from build123d import *

# Parameters (mm, degrees)
EXTRUDE_1_DEPTH = 2
SKETCH_2_R      = 2.5
EXTRUDE_2_DEPTH = 30


with BuildPart() as part:
    # 草图1 → 凸台-拉伸1 (new body)
    with BuildSketch(Plane(origin=(0, 0, 0), x_dir=(1, 0, 0), z_dir=(0, 1, 0))):
        with BuildLine():
            Line((64.772727273, 118.409090909), (138.257575758, 118.409090909))
            Line((138.257575758, 118.409090909), (138.257575758, 143.409090909))
            ThreePointArc((138.257575758, 143.409090909), (141.186507946, 150.480158721), (148.257575758, 153.409090909))
            Line((148.257575758, 153.409090909), (153.257575758, 153.409090909))
            ThreePointArc((153.257575758, 153.409090909), (160.328643569, 150.480158721), (163.257575758, 143.409090909))
            Line((163.257575758, 143.409090909), (163.257575758, 118.409090909))
            Line((163.257575758, 118.409090909), (200, 118.409090909))
            Line((200, 118.409090909), (200, 0))
            Line((200, 0), (0, 0))
            Line((0, 0), (0, 118.409090909))
            Line((0, 118.409090909), (39.772727273, 118.409090909))
            Line((39.772727273, 118.409090909), (39.772727273, 143.409090909))
            ThreePointArc((39.772727273, 143.409090909), (42.701659461, 150.480158721), (49.772727273, 153.409090909))
            Line((49.772727273, 153.409090909), (54.772727273, 153.409090909))
            ThreePointArc((54.772727273, 153.409090909), (61.843795085, 150.480158721), (64.772727273, 143.409090909))
            Line((64.772727273, 143.409090909), (64.772727273, 118.409090909))
        make_face()
    extrude(amount=EXTRUDE_1_DEPTH)

    # 草图2 → 凸台-拉伸2 (add)
    with BuildSketch(Plane(origin=(0, 2, 0), x_dir=(1, 0, 0), z_dir=(0, 1, 0))):
        with Locations(Location((52.11924037, 143.695636013, 0), (0, 0, 90))):
            Circle(SKETCH_2_R)
        with Locations(Location((151.328174324, 143.695636013, 0), (0, 0, 90))):
            Circle(SKETCH_2_R)
    extrude(amount=EXTRUDE_2_DEPTH)


solid = part.part
Could you check a few things on this model? Use its own coordinates, in mm. A direction names the side the tool comes from. Give positions to 0.01 mm unless a question says otherwise; leave off trailing zeros. Order: outer loops, then holes, each group sorted by start corner. A loop starts at its lowest first (then second) coordinate and runs counter-clockwise, first axis right, second up. Notation, with made-up numbers: (69, 5) - (118, 5) arc R19 ccw to (118, 10) - close; hole circle Ø9 at (36.25, 45). An arc over 180 degrees is marked (long way). Return JSON: item names as keys, results as strings. Group by question number.
Q1. Which directions (+Z, -Z, +X, -X, +Y, -Y) give clear straight access to the entire face, cutting with the end or side of a thin tool? Please do faces 1 (the face through (141.11, 0.99, -150.4)), 2 (the face through (53.077, 16.79, -146.005)), 3 (the face through (52, 32, -144)).
Q2. Will these pins go through, and if not, where does the flat tip stop? pin 1 Ø1 at (x, y) = (173.5, 1) entering from -Z; pin 2 Ø12 at (x, z) = (150.5, -77.5) entering from -Y; pin 3 Ø12 at (x, y) = (28, 11) entering from +Z; pin 4 Ø1 at (y, z) = (1, -125.5) entering from -X.
Q3. Suppose I cut it at C-C, the plane x = 184. Please give me the cut outline in (y, z), and give its area (3 significant figures).
Q4. Please list where this line runs through material, in increasing order: line 1 along Y through (x, z) = (9, -46). Write a range as [from, to].
Q5. Suppose I cut it at A-A, the plane y = 19. Please give me the cut outline in (x, z).
Q6. Suppose I cut it at B-B, the plane z = -22. Please give me the cut outline in (x, y), and give its area (3 significant figures).
Q7. Thinking about a two-plate mould opening in X: for faces 4 (the face through (151, 32, -144)), 5 (the face through (61.766, 0.986, -150.557)), 6 (the face through (42.62, 0.99, -150.4)), 7 (the face through (160.25, 0.99, -150.56)), which applies, pulls with the +X half, pulls with the -X half, needs draft (parallel to the pull), parting line crosses it, or undercut?
Resolved:
{
 "1": {"face 1": "-Z, +Y, -Y", "face 2": "+Y", "face 3": "+Z, -Z, +X, -X, +Y"},
 "2": {"pin 1": "stops at z = -118.41", "pin 2": "stops at y = 0", "pin 3": "passes through", "pin 4": "stops at x = 39.77"},
 "3": {"outline": "(0, -118.41) - (2, -118.41) - (2, 0) - (0, 0) - close", "area": "237 mm2"},
 "4": {"line 1": "y = [0, 2]"},
 "5": {"outline": "circle Ø5 at (52.12, -143.7); circle Ø5 at (151.33, -143.7)"},
 "6": {"outline": "(0, 0) - (200, 0) - (200, 2) - (0, 2) - close", "area": "400 mm2"},
 "7": {"face 4": "needs draft", "face 5": "undercut", "face 6": "pulls with the -X half", "face 7": "pulls with the +X half"}
}
